Build history of the part. All positions in model axes, mm. A direction names the side the tool comes from. Round coordinates to 2 decimals unless told otherwise and drop trailing zeros. Write each loop counter-clockwise with the first axis right and the second up, starting at its lowest first coordinate (ties: lowest second). Pieces come first, ordered by that corner, then holes.
1) Saw through at A-A (x = 0). Write the cut outline in (y, z).
2) Saw through at D-D (x = 3). Write the cut outline in (y, z), plus the area to 3 significant figures.
3) Pull direction Y, two halves, no side cores. Call faces 1 (the cylindrical face through (6.466, -2.681, -2.014)), 2 (the cylindrical face through (2.58, 4.05, -2.56)), 3 (the flat face through (-2, 5, 1.5)): +Y half, -Y half, draft (parallel to the pull), parting line (faces both ways), or undercut.
4) Saw through at B-B (y = 5.25). Write the cut outline in (x, z), plus the area to 3 significant figures.
5) Flat gauge pins, fed straight in: pin 1 (1 mm diameter, centred on x = 1.5, z = 0.5, fed in from +Y); pin 2 (1 mm diameter, centred on y = -2.5, z = -1.5, fed in from -X); pin 3 (2.5 mm diameter, centred on x = 1.5, y = 2, fed in from -Z). Where does each tip first touch, or does it go through?
6) Saw through at C-C (z = 0.55). Write the cut outline in (x, y).
7) Wall check: probe 1 along Y at (x, z) = (0, -2.6); probe 2 along Z at (x, y) = (2, 5); probe 3 along Y at (x, z) = (0, 0). Give the ranges that are in metal, low to high.
8) Which spindle directions (+Z, -Z, +X, -X, +Y, -Y) get a long thin tool onto all of the face, cutting with end or side? Do faces 4 (the cylindrical face through (-0.867, -3.905, -0.572)), 5 (the cylindrical face through (-1.08, -4.88, 0.23)), 6 (the flat face through (-2, -5, -3)). Say none if no direction does.
from build123d import *

# Parameters (mm, degrees)
D10_PILOT_AND_M10X0P5_THREAD_ENVELOPE_START = -1
SKETCH1_R                                   = 5
SKETCH1_R_2                                 = 4
D10_PILOT_AND_M10X0P5_THREAD_ENVELOPE_DEPTH = 2
OUTER_RACE_INNER_SHOULDER_ID7P4_START       = 1
SKETCH2_R                                   = 5
SKETCH2_R_2                                 = 3.7
OUTER_RACE_INNER_SHOULDER_ID7P4_DEPTH       = 0.8
INBOARD_G10_RETENTION_FLANGE_H0P3_START     = 1.5
SKETCH3_R                                   = 7
SKETCH3_R_2                                 = 3.7
INBOARD_G10_RETENTION_FLANGE_H0P3_DEPTH     = 0.3
M14X0P5_BEARING_CAP_BOSS_START              = -2.1
SKETCH4_R                                   = 7
SKETCH4_R_2                                 = 4
M14X0P5_BEARING_CAP_BOSS_DEPTH              = 1.1
FLANGED_RACE_POCKET_D9P6_START              = -3
SKETCH5_R                                   = 7
SKETCH5_R_2                                 = 4.8
FLANGED_RACE_POCKET_D9P6_DEPTH              = 0.9


with BuildPart() as part:
    # Sketch1 → D10_Pilot_And_M10x0p5_Thread_Envelope (new body)
    with BuildSketch(Plane.XY.offset(D10_PILOT_AND_M10X0P5_THREAD_ENVELOPE_START)):
        Circle(SKETCH1_R)
        Circle(SKETCH1_R_2, mode=Mode.SUBTRACT)
    extrude(amount=D10_PILOT_AND_M10X0P5_THREAD_ENVELOPE_DEPTH)

    # Sketch2 → Outer_Race_Inner_Shoulder_ID7p4 (add)
    with BuildSketch(Plane.XY.offset(OUTER_RACE_INNER_SHOULDER_ID7P4_START)):
        Circle(SKETCH2_R)
        Circle(SKETCH2_R_2, mode=Mode.SUBTRACT)
    extrude(amount=OUTER_RACE_INNER_SHOULDER_ID7P4_DEPTH)

    # Sketch3 → Inboard_G10_Retention_Flange_H0p3 (add)
    with BuildSketch(Plane.XY.offset(INBOARD_G10_RETENTION_FLANGE_H0P3_START)):
        Circle(SKETCH3_R)
        Circle(SKETCH3_R_2, mode=Mode.SUBTRACT)
    extrude(amount=INBOARD_G10_RETENTION_FLANGE_H0P3_DEPTH)

    # Sketch4 → M14x0p5_Bearing_Cap_Boss (add)
    with BuildSketch(Plane.XY.offset(M14X0P5_BEARING_CAP_BOSS_START)):
        Circle(SKETCH4_R)
        Circle(SKETCH4_R_2, mode=Mode.SUBTRACT)
    extrude(amount=M14X0P5_BEARING_CAP_BOSS_DEPTH)

    # Sketch5 → Flanged_Race_Pocket_D9p6 (add)
    with BuildSketch(Plane.XY.offset(FLANGED_RACE_POCKET_D9P6_START)):
        Circle(SKETCH5_R)
        Circle(SKETCH5_R_2, mode=Mode.SUBTRACT)
    extrude(amount=FLANGED_RACE_POCKET_D9P6_DEPTH)


solid = part.part
Evaluation:
1. outline: (-7, -3) - (-4.8, -3) - (-4.8, -2.1) - (-4, -2.1) - (-4, 1) - (-3.7, 1) - (-3.7, 1.8) - (-7, 1.8) - (-7, 1.5) - (-5, 1.5) - (-5, -1) - (-7, -1) - close; (3.7, 1) - (4, 1) - (4, -2.1) - (4.8, -2.1) - (4.8, -3) - (7, -3) - (7, -1) - (5, -1) - (5, 1.5) - (7, 1.5) - (7, 1.8) - (3.7, 1.8) - close
2. outline: (-6.32, -3) - (-3.75, -3) - (-3.75, -2.1) - (-2.65, -2.1) - (-2.65, 1) - (-2.17, 1) - (-2.17, 1.8) - (-6.32, 1.8) - (-6.32, 1.5) - (-4, 1.5) - (-4, -1) - (-6.32, -1) - close; (2.17, 1) - (2.65, 1) - (2.65, -2.1) - (3.75, -2.1) - (3.75, -3) - (6.32, -3) - (6.32, -1) - (4, -1) - (4, 1.5) - (6.32, 1.5) - (6.32, 1.8) - (2.17, 1.8) - close
2. area: 22.5 mm2
3. face 1: parting line
3. face 2: undercut
3. face 3: draft
4. outline: (-4.63, -3) - (4.63, -3) - (4.63, -1) - (-4.63, -1) - close; (-4.63, 1.5) - (4.63, 1.5) - (4.63, 1.8) - (-4.63, 1.8) - close
4. area: 21.3 mm2
5. pin 1: stops at y = 4.9
5. pin 2: stops at x = -6.71
5. pin 3: stops at z = 1
6. outline: circle Ø10 at (0, 0); hole circle Ø8 at (0, 0)
7. probe 1: y = -7 to -4.8, 4.8 to 7
7. probe 2: z = -3 to -1, 1.5 to 1.8
7. probe 3: y = -5 to -4, 4 to 5
8. face 4: -Z
8. face 5: none
8. face 6: -Z, +X, -X, +Y, -Y
